```python
from build123d import *

# Parameters (mm, degrees)
SKETCH1_W                 = 5.5
SKETCH1_H                 = 7
SHELL1_T                  = -0.25
SHELL1_THICKNESS_2_FACE_R = 5.25
SHELL1_THICKNESS_2_DEPTH  = 0.25
SKETCH6_R                 = 5.5
SKETCH6_R_2               = 4
BOSS_EXTRUDE1_DEPTH       = 0.25
WRAP1_SECTION_W           = 0.25
WRAP1_SECTION_H           = 6.5
WRAP1_ANGLE               = 22.397441082
CIRPATTERN1_COUNT         = 6
SKETCH10_W                = 2.48
SKETCH10_H                = 6.5
BOSS_EXTRUDE2_DEPTH       = 0.25
CIRPATTERN2_COUNT         = 6
CUT_EXTRUDE1_REACH        = 14.692
SKETCH12_R                = 0.75


with BuildPart() as part:
    # Sketch1 → Revolve1 (revolve)
    with BuildSketch(Plane.XY, mode=Mode.PRIVATE) as revolve1_sk:
        with Locations((2.75, 3.5)):
            Rectangle(SKETCH1_W, SKETCH1_H)
    revolve(revolve1_sk.sketch.rotate(Axis((0, 0, 0), (0, 1, 0)), 90), axis=Axis((0, 0, 0), (0, 1, 0)))

    # Shell1
    shell1_openings = [part.faces().sort_by_distance(p)[0] for p in [
        (0, 7, 0),
    ]]
    offset(amount=SHELL1_T, openings=shell1_openings, kind=Kind.INTERSECTION)

    # Shell1 thickness 2 face (on inner face of the shell) → Shell1 thickness 2 (add)
    with BuildSketch(Plane(origin=(0, 0.25, 0), x_dir=(0, 0, -1), z_dir=(0, -1, 0))):
        Circle(SHELL1_THICKNESS_2_FACE_R)
    extrude(amount=-SHELL1_THICKNESS_2_DEPTH)

    # Sketch6 → Boss-Extrude1 (add)
    with BuildSketch(Plane(origin=(0, 7, 0), x_dir=(1, 0, 0), z_dir=(0, 1, 0))):
        with Locations(Location((0, 0, 0), (0, 0, 90))):
            Circle(SKETCH6_R)
        with Locations(Location((0, 0, 0), (0, 0, 270))):
            Circle(SKETCH6_R_2, mode=Mode.SUBTRACT)
    extrude(amount=-BOSS_EXTRUDE1_DEPTH)

    # Wrap1 section (on wrap section) → Wrap1 (revolve, cut)
    with BuildSketch(Plane(origin=(0, 0, 0), x_dir=(0.9062945487659477, 0, 0.42264665014303293), z_dir=(-0.42264665014303293, 0, 0.9062945487659477))):
        with Locations((5.375, 3.5)):
            Rectangle(WRAP1_SECTION_W, WRAP1_SECTION_H)
    wrap1 = revolve(axis=Axis((0, 0, 0), (0, 1, 0)), revolution_arc=WRAP1_ANGLE, mode=Mode.SUBTRACT)

    # CirPattern1: Wrap1 ×6 about axis
    cirpattern1_axis = Axis((0, 0, 0), (0, 1, 0))
    for i in range(1, CIRPATTERN1_COUNT):
        add(wrap1.rotate(cirpattern1_axis, i * 360 / CIRPATTERN1_COUNT), mode=Mode.SUBTRACT)

    # Sketch10 → Boss-Extrude2 (add)
    with BuildSketch(Plane.XY):
        with Locations((-4.26, 3.745038645)):
            Rectangle(SKETCH10_W, SKETCH10_H)
    boss_extrude2 = extrude(amount=-BOSS_EXTRUDE2_DEPTH)

    # CirPattern2: Boss-Extrude2 ×6 about axis
    cirpattern2_axis = Axis((0.026764782, 0, 0.000808926), (0, 1, 0))
    for i in range(1, CIRPATTERN2_COUNT):
        add(boss_extrude2.rotate(cirpattern2_axis, i * 360 / CIRPATTERN2_COUNT))

    # Sketch11 → Revolve3 (revolve)
    with BuildSketch(Plane.XY, mode=Mode.PRIVATE) as revolve3_sk:
        Polygon((-5.5, 0), (0, 0), (0, -3), (-1.5, -3), (-1.5, -0.5), (-5.5, -0.5), align=None)
    revolve(revolve3_sk.sketch.rotate(Axis((0, -3, 0), (0, 1, 0)), 270), axis=Axis((0, -3, 0), (0, 1, 0)))

    # Sketch12 → Cut-Extrude1 (cut, up to next)
    with BuildSketch(Plane.XZ.offset(3), mode=Mode.PRIVATE) as cut_extrude1_sk1:
        with Locations(Location((0, 0, 0), (0, 0, 270))):
            Circle(SKETCH12_R)
    cut_extrude1_tool1 = extrude(cut_extrude1_sk1.sketch, amount=-CUT_EXTRUDE1_REACH, mode=Mode.PRIVATE) & part.part
    add(cut_extrude1_tool1.solids().sort_by_distance((0, -3, 0))[0], mode=Mode.SUBTRACT)


solid = part.part
```
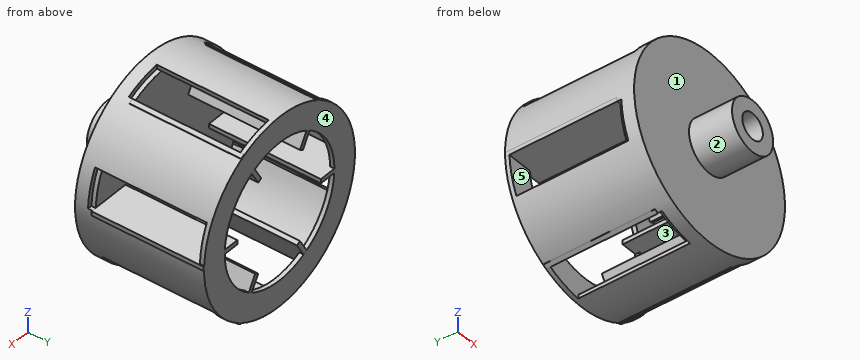
Check sheet for the modelled part. Datum: model origin and axes. Units: mm. Face numbers are marked on the shaded views. A direction names the side the tool comes from. Round coordinates to 2 decimals unless told otherwise and drop trailing zeros. Write each loop counter-clockwise with the first axis right and the second up, starting at its lowest first coordinate (ties: lowest second). Pieces come first, ordered by that corner, then holes. Notation, with made-up numbers: M 87,-30.5 L 116,-30.5 A33 cw 116,-1.5 Z; hole C 44.25,27 d9. An arc over 180 degrees is marked long. Write item = value, one per line. Start each with the question number.
1. Section check D-D, the plane z = 1.75. Record the cut outline in (x, y).
2. Release check for a two-part mould opening along Z. For the marked faces 1, 2 and 3 record: pulls with the +Z half, pulls with the -Z half, needs draft (parallel to the pull), parting line crosses it, or undercut.
3. Section check A-A, the plane x = 0. Record the cut outline in (y, z), then the cut area to 3 significant figures.
4. Tool access check on the marked faces 4 and 5. Record the directions out of +Z, -Z, +X, -X, +Y, -Y that give a thin tool (end or side, any length) a straight path to the whole face; none if there is none.
5. Scan lines: line 1 (X direction, y = -0.9, z = 0); line 2 (X direction, y = -0.3, z = 0); line 3 (Y direction, x = -4.25, z = -2). Record each from-to range of solid material in increasing order. Write a range as [from, to].
6. Gauge pin test, flat ends, axial feed: pin 1 (1.2 mm diameter, centred on x = 0, z = 0, fed in from +Y); pin 2 (1 mm diameter, centred on x = 0.5, z = 4, fed in from -Y); pin 3 (1.5 mm diameter, centred on x = -1, y = -0.5, fed in from -Z); pin 4 (1.5 mm diameter, centred on x = -1, y = 6, fed in from +Z). Record the tip position at first contact, or that the pin passes through.
7. Section check B-B, the plane z = -1. Record the cut outline in (x, y), then the cut area to 3 significant figures.
8. Section check C-C, the plane y = 5.5. State how many separate pieces and enclosed holes the cut face has, then the cut area to 3 significant figures.
Results found:
q1.outline = M -5.21,-0.5 L 5.21,-0.5 L 5.21,0.25 L 4.95,0.25 L 4.95,0.5 L -4.95,0.5 L -4.95,6.75 L -3.6,6.75 L -3.6,7 L -5.21,7 Z; M 3.6,6.75 L 5.21,6.75 L 5.21,7 L 3.6,7 Z
q2.face_1 = needs draft
q2.face_2 = parting line crosses it
q2.face_3 = undercut
q3.outline = M -3,-1.5 L -0.5,-1.5 L -0.5,-5.5 L 7,-5.5 L 7,-4 L 6.75,-4 L 6.75,-5.25 L 0.5,-5.25 L 0.5,-0.75 L -3,-0.75 Z; M -3,0.75 L 0.5,0.75 L 0.5,5.25 L 6.75,5.25 L 6.75,4 L 7,4 L 7,5.5 L -0.5,5.5 L -0.5,1.5 L -3,1.5 Z
q3.area = 17.1 mm^2
q4.face_4 = +Z, -Z, +X, -X, +Y
q4.face_5 = none
q5.line_1 = [-1.5, -0.75], [0.75, 1.5]
q5.line_2 = [-5.5, -0.75], [0.75, 5.5]
q5.line_3 = [-0.5, 0.5], [6.75, 7]
q6.pin_1 = through
q6.pin_2 = -0.5
q6.pin_3 = -5.49
q6.pin_4 = 5.49
q7.outline = M -5.41,-0.5 L -1.12,-0.5 L -1.12,-3 L 1.12,-3 L 1.12,-0.5 L 5.41,-0.5 L 5.41,7 L 3.87,7 L 3.87,6.75 L 5.15,6.75 L 5.15,0.5 L -5.15,0.5 L -5.15,0.25 L -5.41,0.25 Z; M -5.41,6.75 L -3.87,6.75 L -3.87,7 L -5.41,7 Z
q7.area = 18.7 mm^2
q8.separate_pieces = 6
q8.enclosed_holes = 0
q8.area = 8.65 mm^2
